from build123d import *

# Parameters (mm, degrees)
BOSS_EXTRUDE1_DEPTH                       = 74.93
CUT_EXTRUDE1_START                        = -13.499231569
CUT_EXTRUDE1_DEPTH                        = 27.344407223
F_5_32_0_15625_DIAMETER_HOLE1_D           = 3.96875
F_5_32_0_15625_DIAMETER_HOLE1_DEPTH       = 5.08
F_5_32_0_15625_DIAMETER_HOLE1_CSINK_D     = 10.668
F_5_32_0_15625_DIAMETER_HOLE1_CSINK_ANGLE = 100
F_3_8_0_375_DIAMETER_HOLE1_D              = 9.525
F_3_8_0_375_DIAMETER_HOLE1_DEPTH          = 5.08


with BuildPart() as part:
    # Sketch6 → Boss-Extrude1 (new body, symmetric)
    with BuildSketch(Plane.XY):
        with BuildLine():
            Line((0, 0), (0, 5.08))
            Line((0, 5.08), (32.525659605, 5.08))
            ThreePointArc((32.525659605, 5.08), (32.664283789, 5.07873896), (32.80286209, 5.074956256))
            Line((32.80286209, 5.074956256), (65.30699268, 3.891728742))
            Line((65.30699268, 3.891728742), (97.81112327, 2.708501229))
            ThreePointArc((97.81112327, 2.708501229), (97.949609823, 2.702198114), (98.087958789, 2.693376674))
            Line((98.087958789, 2.693376674), (130.527530834, 0.328488024))
            Line((130.527530834, 0.328488024), (162.967102879, -2.036400627))
            ThreePointArc((162.967102879, -2.036400627), (167.673823883, -2.829176028), (172.14912896, -4.488501164))
            Line((172.14912896, -4.488501164), (171.909045825, -7.781761568))
            Line((171.909045825, -7.781761568), (130.158172165, -4.738066444))
            Line((130.158172165, -4.738066444), (97.71860012, -2.373177794))
            ThreePointArc((97.71860012, -2.373177794), (97.672483798, -2.370237314), (97.626321614, -2.368136275))
            Line((97.626321614, -2.368136275), (65.122191024, -1.184908762))
            Line((65.122191024, -1.184908762), (32.618060434, -0.001681248))
            ThreePointArc((32.618060434, -0.001681248), (32.571867667, -0.000420347), (32.525659605, 0))
            Line((32.525659605, 0), (0, 0))
        make_face()
    boss_extrude1 = extrude(amount=BOSS_EXTRUDE1_DEPTH, both=True)

    # Sketch11 → Cut-Extrude1 (cut)
    with BuildSketch(Plane(origin=(0.344497228, 4.725525927, 0), x_dir=(0.997353242, -0.072708399, 0), z_dir=(0.072708399, 0.997353242, 0)).offset(CUT_EXTRUDE1_START)):
        with BuildLine():
            Line((172.019843553, 62.831668461), (172.019843553, -62.831668461))
            Line((172.019843553, -62.831668461), (61.19754378, -34.980240535))
            ThreePointArc((61.19754378, -34.980240535), (33.920641331, 0), (61.19754378, 34.980240535))
            Line((61.19754378, 34.980240535), (172.019843553, 62.831668461))
        make_face()
    cut_extrude1 = extrude(amount=CUT_EXTRUDE1_DEPTH, mode=Mode.SUBTRACT)

    # Mirror1: Boss-Extrude1, Cut-Extrude1 across plane
    add(boss_extrude1.mirror(Plane(origin=(0, 0, 0), x_dir=(0, 0, 1), z_dir=(1, 0, 0))))
    add(cut_extrude1.mirror(Plane(origin=(0, 0, 0), x_dir=(0, 0, 1), z_dir=(1, 0, 0))), mode=Mode.SUBTRACT)

    # 5/32 (0.15625) Diameter Hole1
    with Locations(Plane(origin=(-1.862802154, 0, 42.848601798), x_dir=(1, 0, 0), z_dir=(0, -1, 0))):
        with Locations((1.862802154, -93.648601798), (1.862802154, 7.951398202)):
            CounterSinkHole(F_5_32_0_15625_DIAMETER_HOLE1_D / 2, F_5_32_0_15625_DIAMETER_HOLE1_CSINK_D / 2, depth=F_5_32_0_15625_DIAMETER_HOLE1_DEPTH, counter_sink_angle=F_5_32_0_15625_DIAMETER_HOLE1_CSINK_ANGLE)

    # 3/8 (0.375) Diameter Hole1
    with Locations(Plane(origin=(0, 5.08, 0), x_dir=(1, 0, 0), z_dir=(0, 1, 0))):
        with Locations((0, 0)):
            Hole(F_3_8_0_375_DIAMETER_HOLE1_D / 2, depth=F_3_8_0_375_DIAMETER_HOLE1_DEPTH)


solid = part.part
Source: CAD feature listing. Evaluate the final solid. Frame: model axes, mm. A direction names the side the tool comes from. Round coordinates to 2 decimals unless told otherwise and drop trailing zeros. Write each loop counter-clockwise with the first axis right and the second up, starting at its lowest first coordinate (ties: lowest second). Pieces come first, ordered by that corner, then holes. Notation, with made-up numbers: (-6, -1) - (18, -1) arc R22 cw to (18, 23) - close; hole circle Ø1 at (0.25, -19). An arc over 180 degrees is marked (long way). Use CSV: the item, a comma, the result in double quotes. Start each with the question number.
(1) Material intervals for probe 1 along Z at (x, y) = (0, 4.2); probe 2 along Z at (x, y) = (0, 1.2); probe 3 along Y at (x, z) = (96.5, -56), sorted ascending. Write a range as [from, to].
(2) Cut plane A-A, the plane x = 135. Return loops of the section in (y, z).
(3) First-contact query: pin 1 Ø2 at (x, z) = (19, 29.5) entering from -Y; pin 2 Ø7.5 at (x, z) = (0, 0) entering from -Y; pin 3 Ø5 at (x, z) = (49.5, 47) entering from +Y; pin 4 Ø4.5 at (x, z) = (0, -50.8) entering from -Y. Flat tips, straight axial feed; report the tip coordinate or a pass-through.
(4) Cut plane D-D, the plane z = -40. Return loops of the section in (x, y).
(5) Mould query, pull axis X, two halves, no side actions, for faces 1 (the face through (1.704, 2.674, -52.106)), 2 (the face through (-167.609, -2.812, -67.607)), 3 (the face through (-2.4, 0.2, 74.93)), 4 (the face through (0.279, 2.674, 52.929)). Classes: pulls with the +X half, pulls with the -X half, needs draft (parallel to the pull), parting line crosses it, or undercut.
(6) Cut plane C-C, the plane x = 9. Return loops of the section in (y, z), and give its area (3 significant figures).
(7) Cut plane B-B, the plane z = 0. Return loops of the section in (x, y), and give its area (3 significant figures).
(8) Set-up query: faces 5 (the face through (3.78, 2.5, 2.9)), 6 (the face through (-8, 0, 1)). Return all of +Z, -Z, +X, -X, +Y, -Y with unobstructed straight access to the full face (end or side cutting, diameter ignored); none if empty.
Geometry says:
1,probe 1,"[-74.93, -52.78], [-48.82, -4.76], [4.76, 48.82], [52.78, 74.93]"
1,probe 2,"[-74.93, -54.7], [-46.9, -4.76], [4.76, 46.9], [54.7, 74.93]"
1,probe 3,"[-2.33, 2.76]"
2,outline,"(-5.09, -74.93) - (0, -74.93) - (0, -53.44) - (-5.09, -53.53) - close; (-5.09, 53.53) - (0, 53.44) - (0, 74.93) - (-5.09, 74.93) - close"
3,pin 1,"y = 0"
3,pin 2,"through"
3,pin 3,"y = 4.56"
3,pin 4,"y = 2.59"
4,outline,"(-81.63, 3.3) - (-81.26, -1.77) - (-32.62, 0) arc R2.54 cw to (-32.53, 0) - (32.53, 0) arc R2.54 cw to (32.62, 0) - (81.26, -1.77) - (81.63, 3.3) - (32.8, 5.07) arc R7.62 ccw to (32.53, 5.08) - (-32.53, 5.08) arc R7.62 ccw to (-32.8, 5.07) - close"
5,face 1,"undercut"
5,face 2,"pulls with the -X half"
5,face 3,"needs draft"
5,face 4,"undercut"
6,outline,"(0, -74.93) - (5.08, -74.93) - (5.08, 74.93) - (0, 74.93) - close"
6,area,"761 mm²"
7,outline,"(-34.38, 5.02) - (-34.01, -0.05) - (-32.62, 0) arc R2.54 cw to (-32.53, 0) - (-4.76, 0) - (-4.76, 5.08) - (-32.53, 5.08) arc R7.62 ccw to (-32.8, 5.07) - close; (4.76, 0) - (32.53, 0) arc R2.54 cw to (32.62, 0) - (34.01, -0.05) - (34.38, 5.02) - (32.8, 5.07) arc R7.62 ccw to (32.53, 5.08) - (4.76, 5.08) - close"
7,area,"299 mm²"
8,face 5,"+Y, -Y"
8,face 6,"+Z, -Z, -Y"
